Geometry: final body of the model. Coordinates: model frame, mm. A direction names the side the tool comes from. Round coordinates to 2 decimals unless told otherwise and drop trailing zeros. Loops run counter-clockwise (first coordinate to the right, second up) from the corner with the lowest first, then second, coordinate; pieces in that order, holes last. Notation, with made-up numbers: M 9,14.25 L 48,14.25 A35 ccw 48,53.25 Z; hole C -23.75,2.5 d1. An arc over 180 degrees is marked long. Answer as a JSON object with one key per item and string values.
```python
from build123d import *

# Parameters (mm, degrees)
CORTAR_EXTRUIR1_DEPTH            = 10
TALADRO_DE_MARGEN_PARA_M51_D     = 5.5
CORTAR_EXTRUIR2_DEPTH            = 6
TALADRO_DE_MARGEN_PARA_M31_D     = 3.4
TALADRO_DE_MARGEN_PARA_M31_DEPTH = 5.766394553


with BuildPart() as part:
    # Croquis1 → Revolución1 (revolve)
    with BuildSketch(Plane(origin=(0, 0, 0), x_dir=(0, 0, -1), z_dir=(1, 0, 0)), mode=Mode.PRIVATE) as revoluci_n1_sk:
        Polygon((-5.25, 0), (5.25, 0), (5.25, 9), (3.75, 9), (3.75, 24), (0.75, 24), (0.75, 8.7), (-5.25, 8.7), align=None)
    revolve(revoluci_n1_sk.sketch.rotate(Axis((0, 0, 25.623234534), (0, 0, -1)), 90), axis=Axis((0, 0, 25.623234534), (0, 0, -1)))

    # Croquis2 → Cortar-Extruir1 (cut)
    with BuildSketch(Plane.XY.offset(5.25)):
        with BuildLine():
            Line((-1.8, 2.4), (1.8, 2.4))
            ThreePointArc((1.8, 2.4), (0, -3), (-1.8, 2.4))
        make_face()
    extrude(amount=-CORTAR_EXTRUIR1_DEPTH, mode=Mode.SUBTRACT)

    # Taladro de margen para M51 (through all)
    with Locations(Plane(origin=(0, 17.5, -3.75), x_dir=(-1, 0, 0), z_dir=(0, 0, -1))):
        with Locations((0, 0), (12.374368671, -5.125631329), (17.5, -17.5), (12.374368671, -29.874368671), (0, -35), (-12.374368671, -29.874368671), (-17.5, -17.5), (-12.374368671, -5.125631329)):
            Hole(TALADRO_DE_MARGEN_PARA_M51_D / 2)

    # Croquis10 → Cortar-Extruir2 (cut)
    with BuildSketch(Plane.XY.offset(5.25)):
        with BuildLine():
            Line((-3, 8.166394553), (3, 8.166394553))
            ThreePointArc((3, 8.166394553), (0, 8.7), (-3, 8.166394553))
        make_face()
    extrude(amount=-CORTAR_EXTRUIR2_DEPTH, mode=Mode.SUBTRACT)

    # Taladro de margen para M31
    with Locations(Plane(origin=(0, 8.166394553, 2.25), x_dir=(0, 0, 1), z_dir=(0, 1, 0))):
        with Locations((0, 0)):
            Hole(TALADRO_DE_MARGEN_PARA_M31_D / 2, depth=TALADRO_DE_MARGEN_PARA_M31_DEPTH)


solid = part.part
```
1) Set-up query: faces 1 (the face through (0, -3, 0)), 2 (the face through (-10, 0, -3.75)), 3 (the face through (-0.7, 5.2, 0.7)). Return all of +Z, -Z, +X, -X, +Y, -Y with unobstructed straight access to the full face (end or side cutting, diameter ignored); none if empty.
Geometry results:
{"face 1": "+Z", "face 2": "-Z", "face 3": "+Y"}
2) Cut plane A-A on x = 0. Return the cut outline in (y, z).
Geometry results:
{"outline": "M -24,-3.75 L -20.25,-3.75 L -20.25,-0.75 L -24,-0.75 Z; M -14.75,-3.75 L -9,-3.75 L -9,-5.25 L 9,-5.25 L 9,-3.75 L 14.75,-3.75 L 14.75,-0.75 L 8.17,-0.75 L 8.17,0.55 L 2.4,0.55 L 2.4,-4.75 L -3,-4.75 L -3,5.25 L -8.7,5.25 L -8.7,-0.75 L -14.75,-0.75 Z; M 2.4,3.95 L 8.17,3.95 L 8.17,5.25 L 2.4,5.25 Z; M 20.25,-3.75 L 24,-3.75 L 24,-0.75 L 20.25,-0.75 Z"}
3) Cut plane B-B on y = 1. Return the cut outline in (x, z), and give its area (3 significant figures).
Geometry results:
{"outline": "M -23.98,-3.75 L -20.06,-3.75 L -20.06,-0.75 L -23.98,-0.75 Z; M -14.94,-3.75 L -8.94,-3.75 L -8.94,-5.25 L 8.94,-5.25 L 8.94,-3.75 L 14.94,-3.75 L 14.94,-0.75 L 8.64,-0.75 L 8.64,5.25 L 2.83,5.25 L 2.83,-4.75 L -2.83,-4.75 L -2.83,5.25 L -8.64,5.25 L -8.64,-0.75 L -14.94,-0.75 Z; M 20.06,-3.75 L 23.98,-3.75 L 23.98,-0.75 L 20.06,-0.75 Z", "area": "187 mm2"}
4) Line query: probe 1 along Y at (x, z) = (0, -2.8); probe 2 along X at (y, z) = (0.5, -3.25); probe 3 along Y at (x, z) = (2, -2). Output: solid intervals per line, ascending.
Geometry results:
{"probe 1": "-24 to -20.25, -14.75 to -3, 2.4 to 14.75, 20.25 to 24", "probe 2": "-23.99 to -20.2, -14.8 to -2.96, 2.96 to 14.8, 20.2 to 23.99", "probe 3": "-23.92 to -19.39, -15.61 to -2.24, 2.24 to 15.61, 19.39 to 23.92"}
5) Pull-direction query (X, two-part tool) for faces 4 (the face through (-0.358, 20.227, -2.229)), 5 (the face through (10.348, -10.516, -2.229)), 6 (the face through (0.34, -8.693, 2.292)), 7 (the face through (10, 0, -0.75)); classes: +X half, -X half, draft (parallel to the pull), parting line (faces both ways), or undercut.
Geometry results:
{"face 4": "undercut", "face 5": "undercut", "face 6": "parting line", "face 7": "draft"}
6) First-contact query: pin 1 (5 mm diameter, centred on x = 17.5, y = 13, fed in from +Z); pin 2 (6 mm diameter, centred on x = 0, y = 0, fed in from +Z); pin 3 (1 mm diameter, centred on x = 2.5, z = 3.5, fed in from -Y); pin 4 (3 mm diameter, centred on x = 0.5, z = -1, fed in from -Y). Flat tips, straight axial feed; report the tip coordinate or a pass-through.
Geometry results:
{"pin 1": "z = -0.75", "pin 2": "z = 5.25", "pin 3": "y = -8.47", "pin 4": "y = -24"}
7) Cut plane C-C on x = 19. Return the cut outline in (y, z), and give its area (3 significant figures).
Geometry results:
{"outline": "M -14.66,-3.75 L -2.3,-3.75 L -2.3,-0.75 L -14.66,-0.75 Z; M 2.3,-3.75 L 14.66,-3.75 L 14.66,-0.75 L 2.3,-0.75 Z", "area": "74.1 mm2"}
8) Cut plane D-D on y = -17.5. Return the cut outline in (x, z), and give its area (3 significant figures).
Geometry results:
{"outline": "M -16.42,-3.75 L -2.75,-3.75 L -2.75,-0.75 L -16.42,-0.75 Z; M 2.75,-3.75 L 16.42,-3.75 L 16.42,-0.75 L 2.75,-0.75 Z", "area": "82.0 mm2"}
